```python
from build123d import *

# Parameters (mm, degrees)
SKETCH1_R           = 49.657
BOSS_EXTRUDE1_DEPTH = 3.175
CUT_EXTRUDE1_DEPTH  = 71.297339374
FILLET1_R           = 2.54
FILLET2_R           = 2.54
SKETCH4_R           = 2.54
CUT_EXTRUDE2_DEPTH  = 71.297339374


with BuildPart() as part:
    # Sketch1 → Boss-Extrude1 (new body)
    with BuildSketch(Plane.XY):
        Circle(SKETCH1_R)
    extrude(amount=BOSS_EXTRUDE1_DEPTH)

    # Sketch3 → Cut-Extrude1 (cut, through all)
    with BuildSketch(Plane.XY.offset(3.175)):
        with BuildLine():
            Line((-3.81, 44.41388104), (-3.81, 8.85388104))
            ThreePointArc((-3.81, 8.85388104), (-9.638843783, 0), (-3.81, -8.85388104))
            Line((-3.81, -8.85388104), (-3.81, -44.41388104))
            ThreePointArc((-3.81, -44.41388104), (-44.577, 0), (-3.81, 44.41388104))
        make_face()
        with BuildLine():
            Line((3.81, 8.85388104), (3.81, 44.41388104))
            ThreePointArc((3.81, 44.41388104), (44.577, 0), (3.81, -44.41388104))
            Line((3.81, -44.41388104), (3.81, -8.85388104))
            ThreePointArc((3.81, -8.85388104), (9.638843783, 0), (3.81, 8.85388104))
        make_face()
    extrude(amount=-CUT_EXTRUDE1_DEPTH, mode=Mode.SUBTRACT)

    # Fillet1
    fillet1_edges = [part.edges().sort_by_distance(p)[0] for p in [
        (-3.81, -44.41388104, 1.5875),
        (-3.81, 44.41388104, 1.5875),
        (3.81, 44.41388104, 1.5875),
        (3.81, -44.41388104, 1.5875),
    ]]
    fillet(fillet1_edges, radius=FILLET1_R)

    # Fillet2
    fillet2_edges = [part.edges().sort_by_distance(p)[0] for p in [
        (-3.81, 8.85388104, 1.5875),
        (-3.81, -8.85388104, 1.5875),
        (3.81, -8.85388104, 1.5875),
        (3.81, 8.85388104, 1.5875),
    ]]
    fillet(fillet2_edges, radius=FILLET2_R)

    # Sketch4 → Cut-Extrude2 (cut, through all)
    with BuildSketch(Plane.XY.offset(3.175)):
        Circle(SKETCH4_R)
    extrude(amount=-CUT_EXTRUDE2_DEPTH, mode=Mode.SUBTRACT)


solid = part.part
```
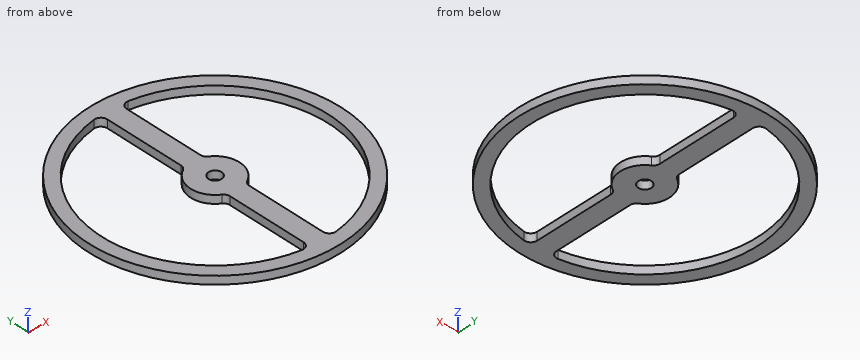
CAD build for the part. Positions are in the model's coordinates, mm. Coordinates: 2 decimals unless noted, no trailing zeros. Write each loop counter-clockwise with the first axis right and the second up, starting at its lowest first coordinate (ties: lowest second). Pieces come first, ordered by that corner, then holes.
(1) Cut at B-B, the plane z = 0.9. List the corners of the cut face in (x, y).
(2) Cut at C-C, the plane y = 0. List the corners of the cut face in (x, z) (3 decimals).
(3) Cut at D-D, the plane y = -17.5. List the corners of the cut face in (x, z) (3 decimals).
(4) Drill centre lines: probe 1 along X at (y, z) = (-28, 1); probe 2 along Y at (x, z) = (0, 1.7); probe 3 along X at (y, z) = (-6, 1.55). Where is each one in solid material? Low to high.
(5) Flat gauge pins, fed straight in: pin 1 (2 mm diameter, centred on x = -35, y = -25, fed in from -Z); pin 2 (1.5 mm diameter, centred on x = -25.5, z = 1, fed in from -Y). Where does each tip first touch, or does it go through?
(6) Cut at A-A, the plane x = 0. List the corners of the cut face in (y, z) (3 decimals), and give its area (3 significant figures).
Geometry says:
1. outline: circle Ø99.31 at (0, 0); hole (-6.73, -44.07) arc R2.54 ccw to (-3.81, -41.55) - (-3.81, -10.39) arc R2.54 ccw to (-5.03, -8.22) arc R9.64 cw to (-5.03, 8.22) arc R2.54 ccw to (-3.81, 10.39) - (-3.81, 41.55) arc R2.54 ccw to (-6.73, 44.07) arc R44.58 ccw to start; hole circle Ø5.08 at (0, 0); hole (3.81, -41.55) arc R2.54 ccw to (6.73, -44.07) arc R44.58 ccw to (6.73, 44.07) arc R2.54 ccw to (3.81, 41.55) - (3.81, 10.39) arc R2.54 ccw to (5.03, 8.22) arc R9.64 cw to (5.03, -8.22) arc R2.54 ccw to (3.81, -10.39) - close
2. outline: (-49.657, 0) - (-44.577, 0) - (-44.577, 3.175) - (-49.657, 3.175) - close; (-9.639, 0) - (-2.54, 0) - (-2.54, 3.175) - (-9.639, 3.175) - close; (2.54, 0) - (9.639, 0) - (9.639, 3.175) - (2.54, 3.175) - close; (44.577, 0) - (49.657, 0) - (49.657, 3.175) - (44.577, 3.175) - close
3. outline: (-46.471, 0) - (-40.998, 0) - (-40.998, 3.175) - (-46.471, 3.175) - close; (-3.81, 0) - (3.81, 0) - (3.81, 3.175) - (-3.81, 3.175) - close; (40.998, 0) - (46.471, 0) - (46.471, 3.175) - (40.998, 3.175) - close
4. probe 1: x = -41.01 to -34.69, -3.81 to 3.81, 34.69 to 41.01
4. probe 2: y = -49.66 to -2.54, 2.54 to 49.66
4. probe 3: x = -49.29 to -44.17, -7.54 to 7.54, 44.17 to 49.29
5. pin 1: passes through
5. pin 2: stops at y = -43.05
6. outline: (-49.657, 0) - (-2.54, 0) - (-2.54, 3.175) - (-49.657, 3.175) - close; (2.54, 0) - (49.657, 0) - (49.657, 3.175) - (2.54, 3.175) - close
6. area: 299 mm2
